Here's how the part is built. I have some questions about the finished solid (model axes, mm). Round coordinates to 2 decimals unless told otherwise and drop trailing zeros. Order: outer loops, then holes, each group sorted by start corner. A loop starts at its lowest first (then second) coordinate and runs counter-clockwise, first axis right, second up.
```python
from build123d import *

# Parameters (mm, degrees)
BOSS_EXTRUDE1_DEPTH     = 3.175
SKETCH3_R               = 2.413
CUT_EXTRUDE1_DEPTH      = 1
CUT_EXTRUDE1_DEPTH_BACK = 4.175


with BuildPart() as part:
    # Sketch1 → Boss-Extrude1 (new body)
    with BuildSketch(Plane.XY):
        with BuildLine():
            Line((0, 50.8), (0, 0))
            Line((0, 0), (103.778975516, 0))
            ThreePointArc((103.778975516, 0), (88.9, 35.921024484), (52.978975516, 50.8))
            Line((52.978975516, 50.8), (0, 50.8))
        make_face()
    extrude(amount=BOSS_EXTRUDE1_DEPTH)

    # Sketch3 → Cut-Extrude1 (cut, two sides)
    with BuildSketch(Plane.XY.offset(3.175)) as cut_extrude1_sk:
        with Locations((64.726475516, 34.925)):
            Circle(SKETCH3_R)
        with Locations((27.896475516, 34.925)):
            Circle(SKETCH3_R)
        with Locations((27.896475516, 15.875)):
            Circle(SKETCH3_R)
        with Locations((64.726475516, 15.875)):
            Circle(SKETCH3_R)
    extrude(amount=CUT_EXTRUDE1_DEPTH, mode=Mode.SUBTRACT)
    extrude(cut_extrude1_sk.sketch, amount=-CUT_EXTRUDE1_DEPTH_BACK, mode=Mode.SUBTRACT)


solid = part.part
```
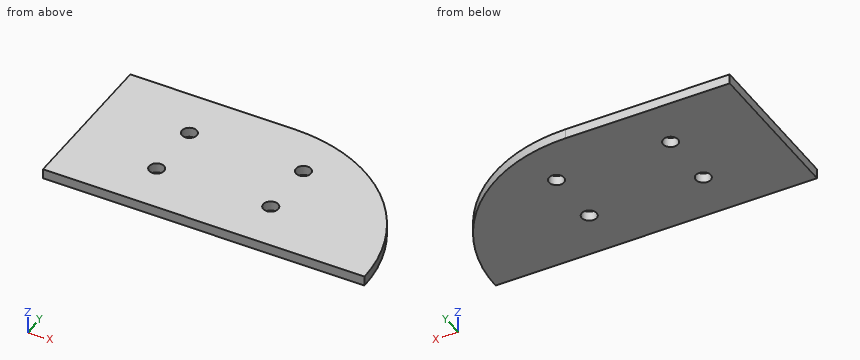
1) If we section it at A-A (y = 33.5): Write out the boundary of the cut face in (x, z) (3 decimals).
2) If we section it at C-C (z = 2.15): Write out the boundary of the cut face in (x, y) (3 decimals).
3) If we section it at B-B (x = 26.5): Write out the boundary of the cut face in (y, z) (3 decimals).
4) I need wall thicknesses on line 1 (X direction, y = 17, z = 2.05); line 2 (X direction, y = 33, z = 2.25); line 3 (Y direction, x = 63, z = 2.9). Which ranges of each line are inside material? Lowest first, please.
5) I'm going to push a flat-ended pin straight in: pin 1 (3 mm diameter, centred on x = 64.73, y = 34.92, fed in from -Z). Where does the tip first touch, or does it pass through?
6) If we section it at D-D (y = 41.5): Write out the boundary of the cut face in (x, z) (3 decimals), plus the area to 3 significant figures.
Solutions:
1. outline: (0, 0) - (25.949, 0) - (25.949, 3.175) - (0, 3.175) - close; (29.844, 0) - (62.779, 0) - (62.779, 3.175) - (29.844, 3.175) - close; (66.674, 0) - (91.168, 0) - (91.168, 3.175) - (66.674, 3.175) - close
2. outline: (0, 0) - (103.779, 0) arc R50.8 ccw to (52.979, 50.8) - (0, 50.8) - close; hole circle Ø4.826 at (27.896, 15.875); hole circle Ø4.826 at (27.896, 34.925); hole circle Ø4.826 at (64.726, 15.875); hole circle Ø4.826 at (64.726, 34.925)
3. outline: (0, 0) - (13.907, 0) - (13.907, 3.175) - (0, 3.175) - close; (17.843, 0) - (32.957, 0) - (32.957, 3.175) - (17.843, 3.175) - close; (36.893, 0) - (50.8, 0) - (50.8, 3.175) - (36.893, 3.175) - close
4. line 1: x = 0 to 25.76, 30.03 to 62.59, 66.86 to 100.85
4. line 2: x = 0 to 26.44, 29.35 to 63.27, 66.18 to 91.6
4. line 3: y = 0 to 14.19, 17.56 to 33.24, 36.61 to 49.8
5. pin 1: passes through
6. outline: (0, 0) - (82.277, 0) - (82.277, 3.175) - (0, 3.175) - close
6. area: 261 mm2
